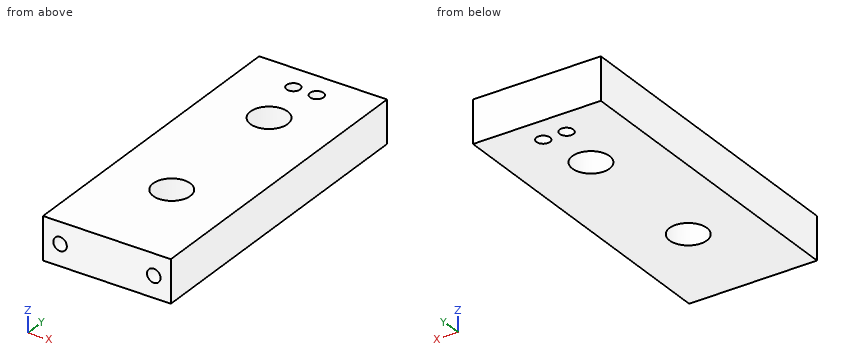
from build123d import *

# Parameters (mm, degrees)
SKETCH1_W                  = 38.1
SKETCH1_H                  = 95.25
SKETCH1_R                  = 5.55625
BOSS_EXTRUDE1_DEPTH        = 12.7
F_10_32_TAPPED_HOLE1_D     = 4.0386
F_10_32_TAPPED_HOLE1_DEPTH = 15.875
F_10_32_TAPPED_HOLE1_TIP   = 1.213317848
F_10_32_TAPPED_HOLE2_D     = 4.0386


with BuildPart() as part:
    # Sketch1 → Boss-Extrude1 (new body)
    with BuildSketch(Plane.XY):
        with Locations((0, 47.625)):
            Rectangle(SKETCH1_W, SKETCH1_H)
        with Locations((0, 28.575)):
            Circle(SKETCH1_R, mode=Mode.SUBTRACT)
        with Locations((0, 71.4375)):
            Circle(SKETCH1_R, mode=Mode.SUBTRACT)
    extrude(amount=BOSS_EXTRUDE1_DEPTH)

    # #10-32 Tapped Hole1
    with Locations(Plane(origin=(0, 0, 0), x_dir=(-1, 0, 0), z_dir=(0, -1, 0))):
        with Locations((13.97, -6.35), (-13.97, -6.35)):
            Hole(F_10_32_TAPPED_HOLE1_D / 2, depth=F_10_32_TAPPED_HOLE1_DEPTH)
            with Locations((0, 0, -(F_10_32_TAPPED_HOLE1_DEPTH + F_10_32_TAPPED_HOLE1_TIP / 2))):  # 118° drill point
                Cone(0, F_10_32_TAPPED_HOLE1_D / 2, F_10_32_TAPPED_HOLE1_TIP, mode=Mode.SUBTRACT)

    # #10-32 Tapped Hole2 (through all)
    with Locations(Plane.XY.offset(12.7)):
        with Locations((-3.4925, 87.3125), (3.4925, 87.3125)):
            Hole(F_10_32_TAPPED_HOLE2_D / 2)


solid = part.part
The model under review builds one solid part; all positions refer to its coordinate system, in mm. Round coordinates to 2 decimals unless told otherwise and drop trailing zeros. Loops run counter-clockwise (first coordinate to the right, second up) from the corner with the lowest first, then second, coordinate; pieces in that order, holes last. Notation, with made-up numbers: (-25, -15.75) -> (15, -15.75) arc R17 cw to (15, -5.75) -> close; hole circle Ø7 at (48, -8). An arc over 180 degrees is marked (long way). Write item = value, one per line. Start each with the question number.
Item 1: Take a section at C-C on z = 2.75. Count the separate pieces of the cut face and the enclosed holes in it, plus the area to 3 significant figures.
Item 2: To check wall thickness, follow L1, parallel to Z at x = -13.97, y = 9; L2, parallel to Y at x = 0, z = 10; L3, parallel to X at y = 87, z = 3. State the ranges of each line that lie inside material, in increasing order.
Item 3: Take a section at D-D on y = 12. Give the boundary of the cut face in (x, z).
Item 4: Take a section at A-A on x = 0. Give the boundary of the cut face in (y, z).
Item 5: Take a section at B-B on y = 67.5. Give the boundary of the cut face in (x, z).
Item 6: Insertion check: pin 1 (10 mm diameter, centred on x = 0, y = 28.575, fed in from +Z); pin 2 (3 mm diameter, centred on x = -13.97, z = 6.35, fed in from -Y). Each pin has a flat end and moves straight along its axis. Give the tip position at first contact, or say it passes through.
Result:
q1.separate_pieces = 1
q1.enclosed_holes = 4
q1.area = 3,410 mm²
q2.L1 = 0 to 4.33, 8.37 to 12.7
q2.L2 = 0 to 23.02, 34.13 to 65.88, 76.99 to 95.25
q2.L3 = -19.05 to -5.49, -1.5 to 1.5, 5.49 to 19.05
q3.outline = (-19.05, 0) -> (19.05, 0) -> (19.05, 12.7) -> (-19.05, 12.7) -> close; hole circle Ø4.04 at (-13.97, 6.35); hole circle Ø4.04 at (13.97, 6.35)
q4.outline = (0, 0) -> (23.02, 0) -> (23.02, 12.7) -> (0, 12.7) -> close; (34.13, 0) -> (65.88, 0) -> (65.88, 12.7) -> (34.13, 12.7) -> close; (76.99, 0) -> (95.25, 0) -> (95.25, 12.7) -> (76.99, 12.7) -> close
q5.outline = (-19.05, 0) -> (-3.92, 0) -> (-3.92, 12.7) -> (-19.05, 12.7) -> close; (3.92, 0) -> (19.05, 0) -> (19.05, 12.7) -> (3.92, 12.7) -> close
q6.pin_1 = through
q6.pin_2 = 16.19
